Autodesk Inventor part; units mm, degrees
ref_plane "YZ Plane" through (0, 0, 0) normal (1, 0, 0) x (0, 1, 0)
ref_plane "XZ Plane" through (0, 0, 0) normal (0, 1, 0) x (-1, 0, 0)
ref_plane "XY Plane" through (0, 0, 0) normal (0, 0, 1) x (1, 0, 0)
sketch "Sketch_19" plane through (0, 0, 0) normal (0, 1, 0) x (-1, 0, 0)
  line L0 (20.2438, -10.5029) -> (20.2438, 10.5029)
  line L1 (20.2438, 10.5029) -> (5, 10.5029)
  arc A0 (5, 10.5029) -> (0, 5.5029) centre (5, 5.5029) ccw
  line L2 (0, 5.5029) -> (0, -5.5029)
  arc A1 (0, -5.5029) -> (5, -10.5029) centre (5, -5.5029) ccw
  line L3 (5, -10.5029) -> (20.2438, -10.5029)
extrude "Extrusion1" add sketch "Sketch_19" along normal blind 22.9918
sketch "Sketch_20" plane through (0, 22.9918, 0) normal (0, 1, 0) x (1, 0, 0)
  line L0 (7, 5.5029) -> (7, -5.5029)
  line L1 (-20.2438, 10.5029) -> (-20.2438, -10.5029)
  line L2 (-20.2438, -10.5029) -> (-5, -10.5029)
  arc A0 (-5, -10.5029) -> (0, -5.5029) centre (-5, -5.5029) ccw
  line L3 (0, -5.5029) -> (0, 5.5029)
  arc A1 (0, 5.5029) -> (-5, 10.5029) centre (-5, 5.5029) ccw
  line L4 (-5, 10.5029) -> (-20.2438, 10.5029)
revolve "Revolution1" add sketch "Sketch_20" angle 90 about axis through (7, 22.9918, -5.5029) along (0, 0, -1)
sketch "Sketch_21" plane through (7, 0, 0) normal (1, 0, 0) x (0, 0, -1)
  arc A0 (-10.5029, 34.9918) -> (-5.5029, 29.9918) centre (-5.5029, 34.9918) ccw
  line L0 (-5.5029, 29.9918) -> (5.5029, 29.9918)
  arc A1 (5.5029, 29.9918) -> (10.5029, 34.9918) centre (5.5029, 34.9918) ccw
  line L1 (10.5029, 34.9918) -> (10.5029, 50.2356)
  line L2 (10.5029, 50.2356) -> (-10.5029, 50.2356)
  line L3 (-10.5029, 50.2356) -> (-10.5029, 34.9918)
extrude "Extrusion2" add sketch "Sketch_21" along normal blind 57.501
sketch "Sketch_22" plane through (64.501, 0, 0) normal (1, 0, 0) x (0, 0, -1)
  line L0 (5.5029, 22.9918) -> (-5.5029, 22.9918)
  arc A0 (-10.5029, 34.9918) -> (-5.5029, 29.9918) centre (-5.5029, 34.9918) ccw
  line L1 (-5.5029, 29.9918) -> (5.5029, 29.9918)
  arc A1 (5.5029, 29.9918) -> (10.5029, 34.9918) centre (5.5029, 34.9918) ccw
  line L2 (10.5029, 34.9918) -> (10.5029, 50.2356)
  line L3 (10.5029, 50.2356) -> (-10.5029, 50.2356)
  line L4 (-10.5029, 50.2356) -> (-10.5029, 34.9918)
revolve "Revolution2" add sketch "Sketch_22" angle 90 about axis through (64.501, 22.9918, -5.5029) along (0, 0, -1)
sketch "Sketch_23" plane through (0, 0, 0) normal (0, 1, 0) x (-1, 0, 0)
  arc A0 (-71.501, 5.5029) -> (-76.501, 10.5029) centre (-76.501, 5.5029) ccw
  line L0 (-76.501, 10.5029) -> (-91.7448, 10.5029)
  line L1 (-91.7448, 10.5029) -> (-91.7448, -10.5029)
  line L2 (-91.7448, -10.5029) -> (-76.501, -10.5029)
  arc A1 (-76.501, -10.5029) -> (-71.501, -5.5029) centre (-76.501, -5.5029) ccw
  line L3 (-71.501, -5.5029) -> (-71.501, 5.5029)
extrude "Extrusion3" add sketch "Sketch_23" along normal blind 22.9918
sketch "Sketch_24" plane through (0, 0, 0) normal (0, 0, 1) x (1, 0, 0)
  line L0 (-32.9438, 71.9836) -> (-32.9438, 0)
  line L1 (-32.9438, 0) -> (-20.2438, 0)
  arc A0 (-18.4912, 13.0048) -> (-20.2438, 0) centre (34.459, -0.7516) ccw
  arc A1 (2.0066, 35.9918) -> (-18.4912, 13.0048) centre (10.8872, 7.4403) ccw
  line L2 (2.0066, 35.9918) -> (69.4944, 35.9918)
  arc A2 (89.9922, 13.0048) -> (69.4944, 35.9918) centre (60.6138, 7.4403) ccw
  arc A3 (91.7448, 0) -> (89.9922, 13.0048) centre (37.042, -0.7516) ccw
  line L3 (91.7448, 0) -> (104.4448, 0)
  line L4 (104.4448, 0) -> (104.4448, 71.9836)
  line L5 (104.4448, 71.9836) -> (-32.9438, 71.9836)
extrude "Extrusion4" cut sketch "Sketch_24" along normal mid plane 42.0116
sketch "Sketch_25" plane through (0, 0, 0) normal (0, 0, 1) x (1, 0, 0)
  line L0 (82.4992, 0) -> (82.4992, 35.9918)
  line L1 (82.4992, 35.9918) -> (87.7492, 35.9918)
  line L2 (87.7492, 35.9918) -> (87.7492, 6)
  line L3 (87.7492, 6) -> (85.7492, 6)
  line L4 (85.7492, 6) -> (85.7492, 0)
  line L5 (85.7492, 0) -> (82.4992, 0)
  line L6 (82.4992, 0) -> (82.4992, 35.9918)
revolve "Revolution3" cut sketch "Sketch_25" angle 360 about axis through (82.4992, 0, 0) along (0, -1, 0)
sketch "Sketch_26" plane through (0, 0, 0) normal (0, 0, 1) x (1, 0, 0)
  line L0 (-10.9982, 0) -> (-10.9982, 35.9918)
  line L1 (-10.9982, 35.9918) -> (-5.7482, 35.9918)
  line L2 (-5.7482, 35.9918) -> (-5.7482, 6)
  line L3 (-5.7482, 6) -> (-7.7482, 6)
  line L4 (-7.7482, 6) -> (-7.7482, 0)
  line L5 (-7.7482, 0) -> (-10.9982, 0)
  line L6 (-10.9982, 0) -> (-10.9982, 35.9918)
revolve "Revolution4" cut sketch "Sketch_26" angle 360 about axis through (-10.9982, 0, 0) along (0, -1, 0)
sketch "Sketch_27" plane through (0, 35.9918, 0) normal (0, 1, 0) x (1, 0, 0)
  line L0 (-32.9438, 23.2029) -> (-32.9438, -7.5)
  line L1 (-32.9438, -7.5) -> (-5, -7.5)
  arc A0 (-5, -7.5) -> (-3, -5.5) centre (-5, -5.5) ccw
  line L2 (-3, -5.5) -> (-3, 5.5)
  arc A1 (-3, 5.5) -> (-5, 7.5) centre (-5, 5.5) ccw
  line L3 (-5, 7.5) -> (-20.2438, 7.5)
  line L4 (-20.2438, 7.5) -> (-20.2438, 10.5029)
  line L5 (-20.2438, 10.5029) -> (91.7448, 10.5029)
  line L6 (91.7448, 10.5029) -> (91.7448, 7.5)
  line L7 (91.7448, 7.5) -> (76.501, 7.5)
  arc A2 (76.501, 7.5) -> (74.501, 5.5) centre (76.501, 5.5) ccw
  line L8 (74.501, 5.5) -> (74.501, -5.5)
  arc A3 (74.501, -5.5) -> (76.501, -7.5) centre (76.501, -5.5) ccw
  line L9 (76.501, -7.5) -> (104.4448, -7.5)
  line L10 (104.4448, -7.5) -> (104.4448, 23.2029)
  line L11 (104.4448, 23.2029) -> (-32.9438, 23.2029)
extrude "Extrusion5" cut sketch "Sketch_27" against normal blind 23
properties part number "2062"
Input: part model. Units: mm. Frame: model coordinates. A direction names the side the tool comes from. Give positions to 0.01 mm unless a question says otherwise; leave off trailing zeros. Order: outer loops, then holes, each group sorted by start corner. A loop starts at its lowest first (then second) coordinate and runs counter-clockwise, first axis right, second up. Notation, with made-up numbers: (50.25, 38) - (84.25, 38) arc R17 cw to (84.25, 64) - close; hole circle Ø1 at (44, 51). An arc over 180 degrees is marked (long way). Use a Markdown table: item, result.
(1) Section query A-A (z = 0). State how many separate pieces and enclosed holes the cut face has, then the cut area to 3 significant figures.
Computed values:
| item | result |
|---|---|
| separate pieces | 3 |
| enclosed holes | 0 |
| area | 864 mm2 |
(2) Section query D-D (x = 20.5). Output: boundary loops of the cut face in (y, z).
Computed values:
| item | result |
|---|---|
| outline | (29.99, -5.5) arc R5 ccw to (34.99, -10.5) - (35.99, -10.5) - (35.99, 10.5) - (34.99, 10.5) arc R5 ccw to (29.99, 5.5) - close |
(3) Access query for faces 1 (the cylindrical face through (2, 27.89, -0.08)), 2 (the cylindrical face through (73.005, 11.335, 9.077)), 3 (the flat face through (-9.1, 12.992, -5.1)), 4 (the cylindrical face through (72.93, 11.33, -9)), 5 (the flat face through (82, 21, 7.5)). Directions: +Z, -Z, +X, -X, +Y, -Y. A direction counts if a zero-diameter tool reaches every point of the face in a straight line with its end or side. Return the directions, or none.
Computed values:
| item | result |
|---|---|
| face 1 | +Z, -Z, -Y |
| face 2 | +Z, -Y |
| face 3 | -X, +Y |
| face 4 | -Z, -Y |
| face 5 | +X, +Y |
(4) Line query: line 1 (Z direction, x = 85, y = 19.5); line 2 (X direction, y = 16, z = 4.5); line 3 (Z direction, x = 82.5, y = 2.5). Output: solid intervals per line, ascending. Write a range as from..to.
Computed values:
| item | result |
|---|---|
| line 1 | z = -10.5..-7.5, 7.5..10.5 |
| line 2 | x = -3..0, 71.5..74.5 |
| line 3 | z = -10.5..-3.25, 3.25..10.5 |
(5) Pin query (flat end, axial travel): pin 1 (5.5 mm diameter, centred on y = 16, z = -1, fed in from -X); pin 2 (9 mm diameter, centred on y = 11, z = -2, fed in from +X); pin 3 (10 mm diameter, centred on y = 12, z = 0.5, fed in from -X). Return the tip coordinate at first contact, or that it passes through.
Computed values:
| item | result |
|---|---|
| pin 1 | stops at x = -3 |
| pin 2 | stops at x = 91.27 |
| pin 3 | stops at x = -19.7 |
(6) Draft query along Z for faces 6 (the flat face through (82.4, 6, -3.4)), 7 (the cylindrical face through (35.35, 31.42, 9)), 8 (the flat face through (79.5, 0, 2.5)), 9 (the cylindrical face through (-1.504, 11.335, -9.077)). Return one class per face: released by +Z, released by -Z, zero draft, split by the parting line, or undercut.
Computed values:
| item | result |
|---|---|
| face 6 | undercut |
| face 7 | released by +Z |
| face 8 | zero draft |
| face 9 | released by -Z |
(7) Section query C-C (y = 20.5). Output: boundary loops of the cut face in (x, z).
Computed values:
| item | result |
|---|---|
| outline | (-16.01, -10.5) - (-5, -10.5) arc R5 ccw to (0, -5.5) - (0, 5.5) arc R5 ccw to (-5, 10.5) - (-16.01, 10.5) - (-16.01, 7.5) - (-5, 7.5) arc R2 cw to (-3, 5.5) - (-3, -5.5) arc R2 cw to (-5, -7.5) - (-16.01, -7.5) - close; (71.5, -5.5) arc R5 ccw to (76.5, -10.5) - (87.51, -10.5) - (87.51, -7.5) - (76.5, -7.5) arc R2 cw to (74.5, -5.5) - (74.5, 5.5) arc R2 cw to (76.5, 7.5) - (87.51, 7.5) - (87.51, 10.5) - (76.5, 10.5) arc R5 ccw to (71.5, 5.5) - close |
(8) Section query B-B (y = 12). Output: boundary loops of the cut face in (x, z).
Computed values:
| item | result |
|---|---|
| outline | (-18.74, -10.5) - (-5, -10.5) arc R5 ccw to (0, -5.5) - (0, 5.5) arc R5 ccw to (-5, 10.5) - (-18.74, 10.5) - close; (71.5, -5.5) arc R5 ccw to (76.5, -10.5) - (90.24, -10.5) - (90.24, 10.5) - (76.5, 10.5) arc R5 ccw to (71.5, 5.5) - close; hole circle Ø10.5 at (-11, 0); hole circle Ø10.5 at (82.5, 0) |
